Could you check a few things on this drawing? It's one solid part, dimensions in mm from its lowest x, y, z. Give positions to 0.01 mm unless a question says otherwise; leave off trailing zeros. Loops run counter-clockwise (first coordinate to the right, second up) from the corner with the lowest first, then second, coordinate; pieces in that order, holes last. Notation, with made-up numbers: (41, 6.25) - (48, 6.25) arc R29 ccw to (48, 29.25) - close; hole circle Ø9 at (62.25, -18.5). An arc over 180 degrees is marked (long way). Use a Markdown table: item, result.
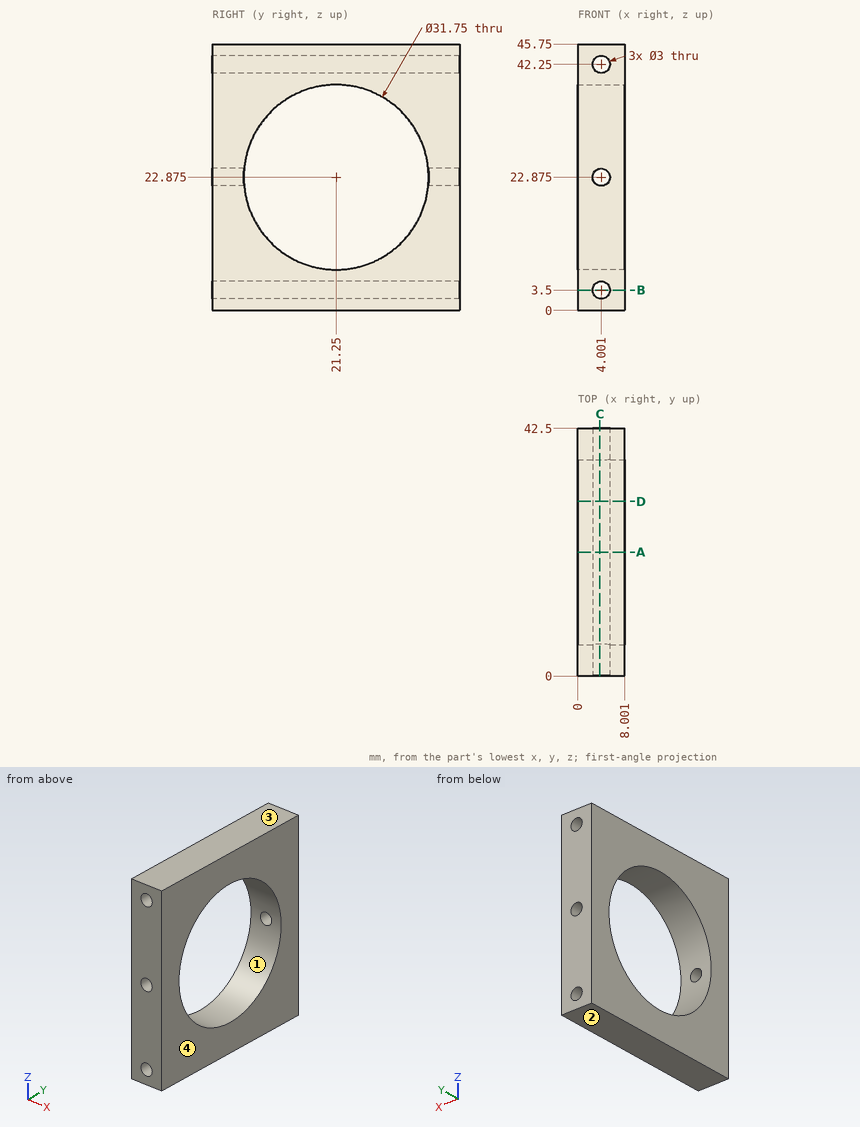
(1) Suppose I cut it at A-A on y = 21.25. Write out the boundary of the cut face in (x, z).
A:
| item | result |
|---|---|
| outline | (0, 0) - (8, 0) - (8, 7) - (0, 7) - close; (0, 38.75) - (8, 38.75) - (8, 45.75) - (0, 45.75) - close; hole circle Ø3 at (4, 3.5); hole circle Ø3 at (4, 42.25) |
(2) Suppose I cut it at D-D on y = 30. Write out the boundary of the cut face in (x, z), plus the area to 3 significant figures.
A:
| item | result |
|---|---|
| outline | (0, 0) - (8, 0) - (8, 9.63) - (0, 9.63) - close; (0, 36.12) - (8, 36.12) - (8, 45.75) - (0, 45.75) - close; hole circle Ø3 at (4, 3.5); hole circle Ø3 at (4, 42.25) |
| area | 140 mm2 |
(3) If I drill on line 1 (X direction, y = 28, z = 42.25); line 2 (Y direction, x = 6.25, z = 21) (1 decimal); line 3 (Y direction, x = 7.5, z = 13), over which ranges is the centre line in solid material (lowest first)?
A:
| item | result |
|---|---|
| line 1 | 0 to 2.5, 5.5 to 8 |
| line 2 | 0 to 5.5, 37 to 42.5 |
| line 3 | 0 to 8.82, 33.68 to 42.5 |
(4) Suppose I cut it at B-B on z = 3.5. Write out the boundary of the cut face in (x, y).
A:
| item | result |
|---|---|
| outline | (0, 0) - (2.5, 0) - (2.5, 42.5) - (0, 42.5) - close; (5.5, 0) - (8, 0) - (8, 42.5) - (5.5, 42.5) - close |
(5) Suppose I cut it at C-C on x = 3.75. Count the separate pieces of the cut face and the enclosed holes in it.
A:
| item | result |
|---|---|
| separate pieces | 4 |
| enclosed holes | 0 |
(6) We'd pull the mould along Z, two halves only. Please class the marked faces 1, 2, 3 and 4: pulls with the +Z half, pulls with the -Z half, needs draft (parallel to the pull), parting line crosses it, or undercut.
A:
| item | result |
|---|---|
| face 1 | undercut |
| face 2 | pulls with the -Z half |
| face 3 | pulls with the +Z half |
| face 4 | needs draft |
